Source: CAD feature listing. Evaluate the final solid. Frame: model axes, mm. A direction names the side the tool comes from. Coordinates: 2 decimals unless noted, no trailing zeros. Write each loop counter-clockwise with the first axis right and the second up, starting at its lowest first coordinate (ties: lowest second). Pieces come first, ordered by that corner, then holes. Notation, with made-up numbers: (-19.75, -27.75) -> (21.25, -27.75) arc R29 ccw to (21.25, 11.25) -> close; hole circle Ø9 at (70.25, -13.75). An arc over 180 degrees is marked (long way). One line per item, written item: value. Start each with the question number.
1. Section query A-A, the plane x = 9. Output: boundary loops of the cut face in (y, z) (3 decimals).
2. Section query B-B, the plane z = -4. Output: boundary loops of the cut face in (x, y).
3. Access query for faces 1 (the flat face through (13, 10, -4)), 2 (the flat face through (21, 5, -1.075)), 3 (the cylindrical face through (8.99, 4.93, -1.075)). Directions: +Z, -Z, +X, -X, +Y, -Y. A direction counts if a zero-diameter tool reaches every point of the face in a straight line with its end or side. Return the directions, or none.
4. First-contact query: P1, Ø3.5, axis at x = 9.5, z = -2.5, coming from the +Y side; P2, Ø2.5, axis at x = 9, z = -3.075, coming from the +Y side. Flat tips, straight axial feed; report the tip coordinate or a pass-through.
5. Mould query, pull axis Z, two halves, no side actions, for faces 4 (the flat face through (13, 5, 1.075)), 5 (the flat face through (13, 2, -7.5)), 6 (the cylindrical face through (10.99, 4.93, -1.075)), 7 (the flat face through (26, 2, -2)). Classes: released by +Z, released by -Z, zero draft, split by the parting line, or undercut.
6. Line query: line 1 (Y direction, x = 18, z = 1); line 2 (Z direction, x = 17.5, y = 8.25) (3 decimals); line 3 (Z direction, x = 11.25, y = 2.25) (3 decimals). Output: solid intervals per line, ascending.
7. Section query C-C, the plane y = 4. State how many separate pieces and enclosed holes the cut face has, and give its area (3 significant figures).
8. Section query D-D, the plane x = 23.75. Output: boundary loops of the cut face in (y, z) (3 decimals).
Autodesk Inventor part; units mm, degrees
ref_plane "YZ Plane" through (0, 0, 0) normal (1, 0, 0) x (0, 1, 0)
ref_plane "XZ Plane" through (0, 0, 0) normal (0, 1, 0) x (-1, 0, 0)
ref_plane "XY Plane" through (0, 0, 0) normal (0, 0, 1) x (1, 0, 0)
sketch "Sketch1" plane through (0, 0, 0) normal (0, 1, 0) x (-1, 0, 0)
  line L0 (0, 0) -> (0, -1.075)
  line L1 (0, 0) -> (0, 1.075) construction
  line L2 (0, -1.075) -> (-26, -1.075) construction
  line L3 (0, 1.075) -> (-26, 1.075)
  line L4 (0, 1.075) -> (0, 7.5) construction
  line L5 (0, -1.075) -> (0, -7.5) construction
  line L6 (-26, -1.075) -> (-26, 1.075)
  line L7 (0, 1.075) -> (0, 7.5)
  line L8 (0, 7.5) -> (-26, 7.5)
  line L9 (-26, 7.5) -> (-26, 1.075)
  line L10 (0, -7.5) -> (-26, -7.5)
  line L11 (-26, -7.5) -> (-26, -1.075)
  line L12 (1, -0.525) -> (1, 1.075) construction
  arc A0 (-1.5221, -0.698) -> (-0.4779, -0.698) centre (-1, -0.525) ccw
  line L13 (0, -0.175) -> (-0.1602, -0.175)
  line L14 (-0.35, -0.3121) -> (-0.4779, -0.698)
  line L15 (-1, -0.525) -> (1, -0.525) construction
  line L16 (0, -0.525) -> (0, -0.175) construction
  arc A1 (-0.1602, -0.175) -> (-0.35, -0.3121) centre (-0.1602, -0.375) ccw
  line L17 (-1, -0.525) -> (-1, 0) construction
  line L18 (-1, -0.525) -> (-1, 0.025) construction
  line L19 (-2, -0.175) -> (-1.8398, -0.175)
  line L20 (-1.65, -0.3121) -> (-1.5221, -0.698)
  arc A2 (-1.65, -0.3121) -> (-1.8398, -0.175) centre (-1.8398, -0.375) ccw
  line L21 (-2, -0.175) -> (-2.1602, -0.175)
  arc A3 (-2.1602, -0.175) -> (-2.35, -0.3121) centre (-2.1602, -0.375) ccw
  line L22 (-2.35, -0.3121) -> (-2.4779, -0.698)
  arc A4 (-3.5221, -0.698) -> (-2.4779, -0.698) centre (-3, -0.525) ccw
  line L23 (-3.65, -0.3121) -> (-3.5221, -0.698)
  arc A5 (-3.65, -0.3121) -> (-3.8398, -0.175) centre (-3.8398, -0.375) ccw
  line L24 (-4, -0.175) -> (-3.8398, -0.175)
  line L25 (-4, -0.175) -> (-4.1602, -0.175)
  arc A6 (-4.1602, -0.175) -> (-4.35, -0.3121) centre (-4.1602, -0.375) ccw
  line L26 (-4.35, -0.3121) -> (-4.4779, -0.698)
  arc A7 (-5.5221, -0.698) -> (-4.4779, -0.698) centre (-5, -0.525) ccw
  line L27 (-5.65, -0.3121) -> (-5.5221, -0.698)
  arc A8 (-5.65, -0.3121) -> (-5.8398, -0.175) centre (-5.8398, -0.375) ccw
  line L28 (-6, -0.175) -> (-5.8398, -0.175)
  line L29 (-6, -0.175) -> (-6.1602, -0.175)
  arc A9 (-6.1602, -0.175) -> (-6.35, -0.3121) centre (-6.1602, -0.375) ccw
  line L30 (-6.35, -0.3121) -> (-6.4779, -0.698)
  arc A10 (-7.5221, -0.698) -> (-6.4779, -0.698) centre (-7, -0.525) ccw
  line L31 (-7.65, -0.3121) -> (-7.5221, -0.698)
  arc A11 (-7.65, -0.3121) -> (-7.8398, -0.175) centre (-7.8398, -0.375) ccw
  line L32 (-8, -0.175) -> (-7.8398, -0.175)
  line L33 (-8, -0.175) -> (-8.1602, -0.175)
  arc A12 (-8.1602, -0.175) -> (-8.35, -0.3121) centre (-8.1602, -0.375) ccw
  line L34 (-8.35, -0.3121) -> (-8.4779, -0.698)
  arc A13 (-9.5221, -0.698) -> (-8.4779, -0.698) centre (-9, -0.525) ccw
  line L35 (-9.65, -0.3121) -> (-9.5221, -0.698)
  arc A14 (-9.65, -0.3121) -> (-9.8398, -0.175) centre (-9.8398, -0.375) ccw
  line L36 (-10, -0.175) -> (-9.8398, -0.175)
  line L37 (-10, -0.175) -> (-10.1602, -0.175)
  arc A15 (-10.1602, -0.175) -> (-10.35, -0.3121) centre (-10.1602, -0.375) ccw
  line L38 (-10.35, -0.3121) -> (-10.4779, -0.698)
  arc A16 (-11.5221, -0.698) -> (-10.4779, -0.698) centre (-11, -0.525) ccw
  line L39 (-11.65, -0.3121) -> (-11.5221, -0.698)
  arc A17 (-11.65, -0.3121) -> (-11.8398, -0.175) centre (-11.8398, -0.375) ccw
  line L40 (-12, -0.175) -> (-11.8398, -0.175)
  line L41 (-12, -0.175) -> (-12.1602, -0.175)
  arc A18 (-12.1602, -0.175) -> (-12.35, -0.3121) centre (-12.1602, -0.375) ccw
  line L42 (-12.35, -0.3121) -> (-12.4779, -0.698)
  arc A19 (-13.5221, -0.698) -> (-12.4779, -0.698) centre (-13, -0.525) ccw
  line L43 (-13.65, -0.3121) -> (-13.5221, -0.698)
  arc A20 (-13.65, -0.3121) -> (-13.8398, -0.175) centre (-13.8398, -0.375) ccw
  line L44 (-14, -0.175) -> (-13.8398, -0.175)
  line L45 (-14, -0.175) -> (-14.1602, -0.175)
  arc A21 (-14.1602, -0.175) -> (-14.35, -0.3121) centre (-14.1602, -0.375) ccw
  line L46 (-14.35, -0.3121) -> (-14.4779, -0.698)
  arc A22 (-15.5221, -0.698) -> (-14.4779, -0.698) centre (-15, -0.525) ccw
  line L47 (-15.65, -0.3121) -> (-15.5221, -0.698)
  arc A23 (-15.65, -0.3121) -> (-15.8398, -0.175) centre (-15.8398, -0.375) ccw
  line L48 (-16, -0.175) -> (-15.8398, -0.175)
  line L49 (-16, -0.175) -> (-16, -1.075) construction
  circle A24 centre (-9, -3.075) radius 1.5
  line L50 (-16, -1.075) -> (-26, -1.075)
  line L51 (0, -1.075) -> (0, -7.5)
  line L52 (-9, -3.075) -> (-9, -1.075) construction
  arc A25 (-17, -1.075) -> (-16.4779, -0.698) centre (-17, -0.525) ccw
  line L53 (-16.35, -0.3121) -> (-16.4779, -0.698)
  arc A26 (-16.1602, -0.175) -> (-16.35, -0.3121) centre (-16.1602, -0.375) ccw
  line L54 (-16, -0.175) -> (-16.1602, -0.175)
  line L55 (0, 0) -> (0, 1.075)
  point P0 (0, -0.5375)
  point P1 (-0.3046, -0.175)
  point P2 (-2.3046, -0.175)
  point P3 (-4.3046, -0.175)
  point P4 (-6.3046, -0.175)
  point P5 (-8.3046, -0.175)
  point P6 (-10.3046, -0.175)
  point P7 (-12.3046, -0.175)
  point P8 (-14.3046, -0.175)
  point P9 (-17.5221, -0.698)
  dimension "d7" = 26
  dimension "d8" = 15
  dimension "d10" = 1.6
  dimension "d12" = 1.1
  dimension "d13" = 2
  dimension "d14" = 1.25
  dimension "d17" = 0.35
  dimension "d18" = 0.2
  dimension "d21" = 2
  dimension "d26" = 3
  dimension "d28" = 2
  dimension "d29" = 9
extrude "Extrusion2" add sketch "Sketch1" along normal blind 10 contours L0 L51 L10 L11 L50 A25 L53 A26 L54 L48 A23 L47 A22 L46 A21 L45 L44 A20 L43 A19 L42 A18 L41 L40 A17 L39 A16 L38 A15 L37 L36 A14 L35 A13 L34 A12 L33 L32 A11 L31 A10 L30 A9 L29 L28 A8 L27 A7 L26 A6 L25 L24 A5 L23 A4 L22 A3 L21 L19 A2 L20 A0 L14 A1 L13 | L3 L9 L8 L7
extrude "Extrusion3" add sketch "Sketch1" against normal blind 5 contours L0 L13 A1 L14 A0 L20 A2 L19 L21 A3 L22 A4 L23 A5 L24 L25 A6 L26 A7 L27 A8 L28 L29 A9 L30 A10 L31 A11 L32 L33 A12 L34 A13 L35 A14 L36 L37 A15 L38 A16 L39 A17 L40 L41 A18 L42 A19 L43 A20 L44 L45 A21 L46 A22 L47 A23 L48 L54 A26 L53 A25 L50 L6 L3 L55 | L0 L51 L10 L11 L50 A25 L53 A26 L54 L48 A23 L47 A22 L46 A21 L45 L44 A20 L43 A19 L42 A18 L41 L40 A17 L39 A16 L38 A15 L37 L36 A14 L35 A13 L34 A12 L33 L32 A11 L31 A10 L30 A9 L29 L28 A8 L27 A7 L26 A6 L25 L24 A5 L23 A4 L22 A3 L21 L19 A2 L20 A0 L14 A1 L13 | L3 L9 L8 L7 | A24
properties part number "Y Axis Carriage"
Computed values:
1. outline: (-5, -7.5) -> (10, -7.5) -> (10, -4.575) -> (0, -4.575) -> (0, -1.575) -> (10, -1.575) -> (10, -1.075) -> (0, -1.075) -> (0, 1.075) -> (10, 1.075) -> (10, 7.5) -> (-5, 7.5) -> close
2. outline: (0, -5) -> (26, -5) -> (26, 10) -> (10.18, 10) -> (10.18, 0) -> (7.82, 0) -> (7.82, 10) -> (0, 10) -> close
3. face 1: +Z, -Z, +X, -X, +Y
3. face 2: +X, +Y
3. face 3: +Y
4. P1: stops at y = 10
4. P2: stops at y = 0
5. face 4: undercut
5. face 5: released by -Z
5. face 6: undercut
5. face 7: zero draft
6. line 1: y = -5 to 0
6. line 2: z = -7.5 to -1.075, 1.075 to 7.5
6. line 3: z = -7.5 to -1.015, 1.075 to 7.5
7. separate pieces: 2
7. enclosed holes: 1
7. area: 334 mm²
8. outline: (-5, -7.5) -> (10, -7.5) -> (10, -1.075) -> (0, -1.075) -> (0, 1.075) -> (10, 1.075) -> (10, 7.5) -> (-5, 7.5) -> close
